Model file for the job. Use its own axes, mm. Round coordinates to 2 decimals unless told otherwise and drop trailing zeros. Order: outer loops, then holes, each group sorted by start corner. A loop starts at its lowest first (then second) coordinate and runs counter-clockwise, first axis right, second up. Notation, with made-up numbers: M 5,9 L 32,9 A21 ccw 32,18 Z; hole C 83,32 d1. An arc over 180 degrees is marked long. Return JSON: item names as keys, results as strings. Group by question number.
Item 1: Slice it at A-A on z = 41.5. Write the cut outline in (x, y).
Item 2: Slice it at D-D on y = 0.6. Give the number of separate pieces and of enclosed holes in the cut face, then the cut area to 3 significant figures.
Item 3: Slice it at B-B on x = 54. Write the cut outline in (y, z).
Item 4: Probe line 1 along X through (y, z) = (1.3, 25); line 2 along Z through (x, y) = (85, 1.5); line 3 along X through (y, z) = (1.25, -10). List the from-to ranges inside material, lowest first.
Item 5: Pin check, flat tip, straight feed: pin 1 Ø0.6 at (x, y) = (99.5, 1) entering from +Z. Stop position of the tip, or through.
Item 6: Pull direction Z, two halves, no side cores. Call faces 1 (the face through (138, 1, -53)), 2 (the face through (-118.306, 1.014, -24.587)), 3 (the face through (13.02, 0.99, 65.37)): pulls with the +Z half, pulls with the -Z half, needs draft (parallel to the pull), parting line crosses it, or undercut.
Item 7: Slice it at C-C on x = -16. Write the cut outline in (y, z), then the cut area to 3 significant figures.
from build123d import *

# Parameters (mm, degrees)
SALIENTE_EXTRUIR1_DEPTH = 2
CROQUIS_BARRENOS_R      = 1.5
CROQUIS_BARRENOS_R_2    = 1
CROQUIS_BARRENOS_R_3    = 0.75
CROQUIS_BARRENOS_R_4    = 1.25
CROQUIS_BARRENOS_R_5    = 2.5
CROQUIS_BARRENOS_R_6    = 3.172
CROQUIS_BARRENOS_W      = 38.6
CROQUIS_BARRENOS_H      = 12.6
CROQUIS_BARRENOS_W_2    = 20
CROQUIS_BARRENOS_H_2    = 25
CROQUIS_BARRENOS_W_3    = 26
CROQUIS_BARRENOS_H_3    = 40
CORTAR_EXTRUIR1_DEPTH   = 159.836393815
REDONDEO1_R             = 3
CHAFL_N2_SIZE           = 5


with BuildPart() as part:
    # Croquis base → Saliente-Extruir1 (new body)
    with BuildSketch(Plane(origin=(0, 0, 0), x_dir=(1, 0, 0), z_dir=(0, 1, 0))):
        Polygon((-140, 75), (-25, 75), (50, 56), (140, 56), (140, -56), (50, -56), (-25, -75), (-140, -75), align=None)
    extrude(amount=SALIENTE_EXTRUIR1_DEPTH)

    # Croquis barrenos → Cortar-Extruir1 (cut, through all)
    with BuildSketch(Plane(origin=(0, 2, 0), x_dir=(1, 0, 0), z_dir=(0, 1, 0))):
        with Locations(Location((-125, -70, 0), (0, 0, 270))):
            Circle(CROQUIS_BARRENOS_R)
        with Locations(Location((-35, -70, 0), (0, 0, 270))):
            Circle(CROQUIS_BARRENOS_R)
        with Locations(Location((85, -50, 0), (0, 0, 270))):
            Circle(CROQUIS_BARRENOS_R)
        with Locations(Location((135, -50, 0), (0, 0, 270))):
            Circle(CROQUIS_BARRENOS_R)
        with Locations(Location((-134.5, -10, 0), (0, 0, 270))):
            Circle(CROQUIS_BARRENOS_R)
        with Locations(Location((-90, -12, 0), (0, 0, 270))):
            Circle(CROQUIS_BARRENOS_R_2)
        with Locations(Location((-64, -12, 0), (0, 0, 270))):
            Circle(CROQUIS_BARRENOS_R_2)
        with Locations(Location((-101.7, -53.446, 0), (0, 0, 270))):
            Circle(CROQUIS_BARRENOS_R_3)
        with Locations(Location((-101.7, -65.446, 0), (0, 0, 270))):
            Circle(CROQUIS_BARRENOS_R_3)
        with Locations(Location((-59.7, -53.446, 0), (0, 0, 270))):
            Circle(CROQUIS_BARRENOS_R_3)
        with Locations(Location((-59.7, -65.446, 0), (0, 0, 270))):
            Circle(CROQUIS_BARRENOS_R_3)
        with Locations(Location((-30, -29, 0), (0, 0, 270))):
            Circle(CROQUIS_BARRENOS_R_4)
        with Locations(Location((19, -29, 0), (0, 0, 270))):
            Circle(CROQUIS_BARRENOS_R_4)
        with Locations(Location((75.075943872, -24.926, 0), (0, 0, 270))):
            Circle(CROQUIS_BARRENOS_R)
        with Locations(Location((124.926, -24.926, 0), (0, 0, 270))):
            Circle(CROQUIS_BARRENOS_R)
        with Locations(Location((107, -25, 0), (0, 0, 270))):
            Circle(CROQUIS_BARRENOS_R)
        with Locations(Location((115, -25, 0), (0, 0, 270))):
            Circle(CROQUIS_BARRENOS_R)
        with Locations(Location((115, -30, 0), (0, 0, 270))):
            Circle(CROQUIS_BARRENOS_R)
        with Locations(Location((107, -30, 0), (0, 0, 270))):
            Circle(CROQUIS_BARRENOS_R)
        with Locations(Location((-45, -35, 0), (0, 0, 270))):
            Circle(CROQUIS_BARRENOS_R_5)
        with Locations(Location((-115.161, -25, 0), (0, 0, 270))):
            Circle(CROQUIS_BARRENOS_R_6)
        with Locations(Location((135, 50, 0), (0, 0, 90))):
            Circle(CROQUIS_BARRENOS_R)
        with Locations(Location((85, 50, 0), (0, 0, 90))):
            Circle(CROQUIS_BARRENOS_R)
        with Locations(Location((124.926, 24.926, 0), (0, 0, 90))):
            Circle(CROQUIS_BARRENOS_R)
        with Locations(Location((115, 30, 0), (0, 0, 90))):
            Circle(CROQUIS_BARRENOS_R)
        with Locations(Location((115, 25, 0), (0, 0, 90))):
            Circle(CROQUIS_BARRENOS_R)
        with Locations(Location((107, 25, 0), (0, 0, 90))):
            Circle(CROQUIS_BARRENOS_R)
        with Locations(Location((107, 30, 0), (0, 0, 90))):
            Circle(CROQUIS_BARRENOS_R)
        with Locations(Location((75.075943872, 24.926, 0), (0, 0, 90))):
            Circle(CROQUIS_BARRENOS_R)
        with Locations(Location((-90, 12, 0), (0, 0, 90))):
            Circle(CROQUIS_BARRENOS_R_2)
        with Locations(Location((-59.7, 65.446, 0), (0, 0, 90))):
            Circle(CROQUIS_BARRENOS_R_3)
        with Locations(Location((-59.7, 53.446, 0), (0, 0, 90))):
            Circle(CROQUIS_BARRENOS_R_3)
        with Locations(Location((-101.7, 53.446, 0), (0, 0, 90))):
            Circle(CROQUIS_BARRENOS_R_3)
        with Locations(Location((-101.7, 65.446, 0), (0, 0, 90))):
            Circle(CROQUIS_BARRENOS_R_3)
        with Locations(Location((19, 29, 0), (0, 0, 90))):
            Circle(CROQUIS_BARRENOS_R_4)
        with Locations(Location((-30, 29, 0), (0, 0, 90))):
            Circle(CROQUIS_BARRENOS_R_4)
        with Locations(Location((-64, 12, 0), (0, 0, 90))):
            Circle(CROQUIS_BARRENOS_R_2)
        with Locations(Location((-45, 35, 0), (0, 0, 90))):
            Circle(CROQUIS_BARRENOS_R_5)
        with Locations(Location((-35, 70, 0), (0, 0, 90))):
            Circle(CROQUIS_BARRENOS_R)
        with Locations(Location((-125, 70, 0), (0, 0, 90))):
            Circle(CROQUIS_BARRENOS_R)
        with Locations(Location((-115.161, 25, 0), (0, 0, 90))):
            Circle(CROQUIS_BARRENOS_R_6)
        with Locations(Location((-134.5, 10, 0), (0, 0, 90))):
            Circle(CROQUIS_BARRENOS_R)
        with Locations((-80.7, -59.446)):
            Rectangle(CROQUIS_BARRENOS_W, CROQUIS_BARRENOS_H)
        with Locations((-21, -49.5)):
            Rectangle(CROQUIS_BARRENOS_W_2, CROQUIS_BARRENOS_H_2)
        with Locations((57, 0)):
            Rectangle(CROQUIS_BARRENOS_W_3, CROQUIS_BARRENOS_H_3)
        with Locations((-80.7, 59.446)):
            Rectangle(CROQUIS_BARRENOS_W, CROQUIS_BARRENOS_H)
        with Locations((-21, 49.5)):
            Rectangle(CROQUIS_BARRENOS_W_2, CROQUIS_BARRENOS_H_2)
    extrude(amount=-CORTAR_EXTRUIR1_DEPTH, mode=Mode.SUBTRACT)

    # Redondeo1
    redondeo1_edges = [part.edges().sort_by_distance(p)[0] for p in [
        (-140, 1, -75),
        (-140, 1, 75),
    ]]
    fillet(redondeo1_edges, radius=REDONDEO1_R)

    # Chaflán2
    chafl_n2_edges = [part.edges().sort_by_distance(p)[0] for p in [
        (140, 1, -56),
        (140, 1, 56),
    ]]
    chamfer(chafl_n2_edges, length=CHAFL_N2_SIZE)


solid = part.part
Output values:
{
 "1": {"outline": "M -140,0 L -31,0 L -31,2 L -140,2 Z; M -11,0 L 140,0 L 140,2 L -11,2 Z"},
 "2": {"separate pieces": "1", "enclosed holes": "47", "area": "33,800 mm²"},
 "3": {"outline": "M 0,-56 L 2,-56 L 2,-20 L 0,-20 Z; M 0,20 L 2,20 L 2,56 L 0,56 Z"},
 "4": {"line 1": "-140 to -118.33, -111.99 to 73.58, 76.57 to 105.5, 108.5 to 113.5, 116.5 to 123.43, 126.42 to 140", "line 2": "-56 to -51.5, -48.5 to 48.5, 51.5 to 56", "line 3": "-140 to -136, -133 to 44, 70 to 140"},
 "5": {"pin 1": "z = 56"},
 "6": {"face 1": "pulls with the -Z half", "face 2": "undercut", "face 3": "pulls with the +Z half"},
 "7": {"outline": "M 0,-72.72 L 2,-72.72 L 2,-62 L 0,-62 Z; M 0,-37 L 2,-37 L 2,37 L 0,37 Z; M 0,62 L 2,62 L 2,72.72 L 0,72.72 Z", "area": "191 mm²"}
}
